Verification items for the finished model (mm, model axes). Give positions to 0.01 mm unless a question says otherwise; leave off trailing zeros. Loops run counter-clockwise (first coordinate to the right, second up) from the corner with the lowest first, then second, coordinate; pieces in that order, holes last. Notation, with made-up numbers: (15.5, -18.5) - (31.5, -18.5) arc R14 ccw to (31.5, 4.5) - close; hole circle Ø2 at (22.25, 50.25). An arc over 180 degrees is marked (long way). Use one line per item in the form item = value.
```python
from build123d import *

# Parameters (mm, degrees)
F0_W     = 69
F0_H     = 69
F1_DEPTH = 25
F2_R     = 10
F3_R     = 10


with BuildPart() as f1:
    # F0 (on Top) → F1 (new body)
    with BuildSketch(Plane.XY):
        with BuildLine():
            Line((100, 66.5), (60, 106.5))
            Line((60, 106.5), (-100, 106.5))
            Line((-100, 106.5), (-100, -40.097934))
            ThreePointArc((-100, -40.097934), (-72.843769, -42.046339), (-46, -37.5))
            ThreePointArc((-46, -37.5), (2.288213, -8.788213), (31, 39.5))
            Line((31, 39.5), (100, 39.5))
            Line((100, 39.5), (100, 63.5))
            Line((100, 63.5), (100, 66.5))
        make_face()
        with BuildLine():
            ThreePointArc((31, 39.5), (2.288213, -8.788213), (-46, -37.5))
            Line((-46, -37.5), (-46, -106.5))
            Line((-46, -106.5), (31, -106.5))
            Line((31, -106.5), (31, -37.5))
            Line((31, -37.5), (100, -37.5))
            Line((100, -37.5), (100, 39.5))
            Line((100, 39.5), (31, 39.5))
        make_face()
        with BuildLine():
            ThreePointArc((-46, -37.5), (-72.843769, -42.046339), (-100, -40.097934))
            Line((-100, -40.097934), (-100, -66.5))
            Line((-100, -66.5), (-60, -106.5))
            Line((-60, -106.5), (-46, -106.5))
            Line((-46, -106.5), (-46, -37.5))
        make_face()
        with Locations((65.5, -72)):
            Rectangle(F0_W, F0_H)
    extrude(amount=F1_DEPTH)

    # F2
    f2_edges = [f1.edges().sort_by_distance(p)[0] for p in [
        (-100, 106.5, 12.5),
    ]]
    fillet(f2_edges, radius=F2_R)

    # F3
    f3_edges = [f1.edges().sort_by_distance(p)[0] for p in [
        (100, -106.5, 12.5),
    ]]
    fillet(f3_edges, radius=F3_R)


solid = f1.part
```
1. Section check A-A, the plane z = 19.25. Record the cut outline in (x, y).
Result set:
outline = (-100, -66.5) - (-60, -106.5) - (90, -106.5) arc R10 ccw to (100, -96.5) - (100, 66.5) - (60, 106.5) - (-90, 106.5) arc R10 ccw to (-100, 96.5) - close
2. Section check B-B, the plane y = 83. Record the cut outline in (x, z), then the cut area to 3 significant figures.
Result set:
outline = (-100, 0) - (83.5, 0) - (83.5, 25) - (-100, 25) - close
area = 4,590 mm²
3. Section check C-C, the plane x = -66. Record the cut outline in (y, z), then the cut area to 4 significant figures.
Result set:
outline = (-100.5, 0) - (106.5, 0) - (106.5, 25) - (-100.5, 25) - close
area = 5,175 mm²
4. Scan lines: probe 1 along X at (y, z) = (82, 1.5); probe 2 along X at (y, z) = (95.5, 14.25); probe 3 along Y at (x, z) = (-82, 21.25). Record each from-to range of solid material in increasing order.
Result set:
probe_1 = -100 to 84.5
probe_2 = -100 to 71
probe_3 = -84.5 to 106.5
